Check sheet for the modelled part. Datum: model origin and axes. Units: mm. Give positions to 0.01 mm unless a question says otherwise; leave off trailing zeros. Loops run counter-clockwise (first coordinate to the right, second up) from the corner with the lowest first, then second, coordinate; pieces in that order, holes last.
```python
from build123d import *

# Parameters (mm, degrees)
F0_W     = 76.2
F0_H     = 19.05
F1_DEPTH = 9.525
F2_R     = 6.35
F3_R     = 5.08


with BuildPart() as f1:
    # F0 (on Front) → F1 (new body, symmetric)
    with BuildSketch(Plane.XZ):
        with Locations((38.1, 2.162681)):
            Rectangle(F0_W, F0_H)
    extrude(amount=F1_DEPTH, both=True)

    # F2
    f2_edges = [f1.edges().sort_by_distance(p)[0] for p in [
        (38.1, 9.525, 11.687681),
        (38.1, -9.525, 11.687681),
        (38.1, -9.525, -7.362319),
        (38.1, 9.525, -7.362319),
    ]]
    fillet(f2_edges, radius=F2_R)

    # F3
    f3_edges = [f1.edges().sort_by_distance(p)[0] for p in [
        (76.2, 0, 11.687681),
    ]]
    fillet(f3_edges, radius=F3_R)


solid = f1.part
```
(1) Gauge pin test, flat ends, axial feed: pin 1 Ø2 at (x, z) = (57.5, -5.5) entering from +Y; pin 2 Ø1.5 at (x, y) = (18.5, -5.5) entering from -Z. Record the tip position at first contact, or that the pin passes through.
(2) Material ranges on line 1 (X direction, y = 5, z = -4.75); line 2 (X direction, y = 0.5, z = 7); line 3 (Z direction, x = 33.5, y = -4.5), recorded low to high.
(3) Section check A-A on x = 53. Record the boundary of the cut face in (y, z) (3 decimals).
Computed values:
1. pin 1: stops at y = 8.48
1. pin 2: stops at z = -7.16
2. line 1: x = 0 to 75.3
2. line 2: x = 0 to 76.18
2. line 3: z = -7.22 to 11.55
3. outline: (-9.525, -1.012) arc R6.35 ccw to (-3.175, -7.362) - (3.175, -7.362) arc R6.35 ccw to (9.525, -1.012) - (9.525, 5.338) arc R6.35 ccw to (3.175, 11.688) - (-3.175, 11.688) arc R6.35 ccw to (-9.525, 5.338) - close
